Part model, mm, in its own coordinate system. Face numbers are marked on the shaded views. A direction names the side the tool comes from. Give positions to 0.01 mm unless a question says otherwise; leave off trailing zeros. Write each loop counter-clockwise with the first axis right and the second up, starting at its lowest first coordinate (ties: lowest second). Pieces come first, ordered by that corner, then holes. Notation, with made-up numbers: M -34.75,-35.75 L -12.75,-35.75 A8 cw -12.75,-29.75 Z; hole C -22,41.25 d10. An arc over 180 degrees is marked long. Use CSV: the item, a comma, the result in double quotes. Start each with the question number.
Item 1: Mould opens along Y. For the marked faces 5, 6 and 7 say: released by +Y, released by -Y, zero draft, split by the parting line, or undercut.
Item 2: Drill centre lines: line 1 (Y direction, x = 21, z = -1.5); line 2 (Y direction, x = 14, z = -4.5); line 3 (Z direction, x = -1, y = 18.25). Where is each one in solid material? Low to high. Write a range as [from, to].
Item 3: Cut at C-C (y = 2.75). List the corners of the cut face in (x, z).
Item 4: Which spindle directions (+Z, -Z, +X, -X, +Y, -Y) get a long thin tool onto all of the face, cutting with end or side? Do the marked faces 1, 2, 3 and 4. Say none if no direction does.
Item 5: Cut at D-D (x = -7.5). List the corners of the cut face in (y, z).
Item 6: Cut at A-A (x = 21.5). List the corners of the cut face in (y, z).
Item 7: Pin check, flat tips, straight feed: pin 1 (0.5 mm diameter, centred on x = 36.5, z = -1.5, fed in from -Y); pin 2 (3 mm diameter, centred on x = 16, z = -7, fed in from -Y); pin 3 (4 mm diameter, centred on x = 3, y = 21.5, fed in from -Z). Stop position of each tip, or through.
Item 8: Cut at B-B (y = 18.25). List the corners of the cut face in (x, z), then the cut area to 3 significant figures.
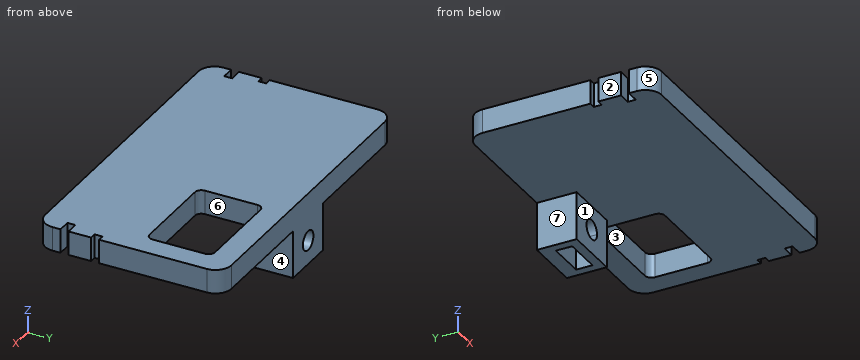
from build123d import *

# Parameters (mm, degrees)
BOSS_EXTRUDE1_DEPTH = 3.81
SKETCH2_W           = 8.89
SKETCH2_H           = 6.35
BOSS_EXTRUDE2_DEPTH = 7.62
CUT_EXTRUDE1_DEPTH  = 7.62
SKETCH4_W           = 6
SKETCH4_H           = 1.674510172
SKETCH4_H_2         = 0.925489708
CUT_EXTRUDE2_DEPTH  = 7.62


with BuildPart() as part:
    # Sketch1 → Boss-Extrude1 (new body)
    with BuildSketch(Plane.XY):
        with BuildLine():
            Line((37.128754647, 0.913367565), (37.128754647, 2.183367565))
            Line((37.128754647, 2.183367565), (35.096754647, 2.183367565))
            Line((35.096754647, 2.183367565), (35.096754647, 3.453367565))
            Line((35.096754647, 3.453367565), (37.128754647, 3.453367565))
            Line((37.128754647, 3.453367565), (37.128754647, 7.053367565))
            Line((37.128754647, 7.053367565), (36.112754647, 7.053367565))
            Line((36.112754647, 7.053367565), (36.112754647, 8.323367565))
            Line((36.112754647, 8.323367565), (37.128754647, 8.323367565))
            Line((37.128754647, 8.323367565), (37.128754647, 25.468367565))
            ThreePointArc((37.128754647, 25.468367565), (36.384805872, 27.264418789), (34.588754647, 28.008367565))
            Line((34.588754647, 28.008367565), (-10.750245353, 28.008367565))
            ThreePointArc((-10.750245353, 28.008367565), (-12.546296577, 27.264418789), (-13.290245353, 25.468367565))
            Line((-13.290245353, 25.468367565), (-13.290245353, 8.323367565))
            Line((-13.290245353, 8.323367565), (-12.274245353, 8.323367565))
            Line((-12.274245353, 8.323367565), (-12.274245353, 7.053367565))
            Line((-12.274245353, 7.053367565), (-13.290245353, 7.053367565))
            Line((-13.290245353, 7.053367565), (-13.290245353, 3.453367565))
            Line((-13.290245353, 3.453367565), (-11.258245353, 3.453367565))
            Line((-11.258245353, 3.453367565), (-11.258245353, 2.183367565))
            Line((-11.258245353, 2.183367565), (-13.290245353, 2.183367565))
            Line((-13.290245353, 2.183367565), (-13.290245353, 0.913367565))
            ThreePointArc((-13.290245353, 0.913367565), (-12.546296577, -0.882683659), (-10.750245353, -1.626632435))
            Line((-10.750245353, -1.626632435), (34.588754647, -1.626632435))
            ThreePointArc((34.588754647, -1.626632435), (36.384805872, -0.882683659), (37.128754647, 0.913367565))
        make_face()
        with BuildLine():
            Line((32.505954647, 24.279567565), (19.094754647, 24.279567565))
            ThreePointArc((19.094754647, 24.279567565), (18.376334158, 23.981988055), (18.078754647, 23.263567565))
            Line((18.078754647, 23.263567565), (18.078754647, 14.881567565))
            ThreePointArc((18.078754647, 14.881567565), (18.376334158, 14.163147076), (19.094754647, 13.865567565))
            Line((19.094754647, 13.865567565), (32.505954647, 13.865567565))
            ThreePointArc((32.505954647, 13.865567565), (33.224375137, 14.163147076), (33.521954647, 14.881567565))
            Line((33.521954647, 14.881567565), (33.521954647, 23.263567565))
            ThreePointArc((33.521954647, 23.263567565), (33.224375137, 23.981988055), (32.505954647, 24.279567565))
        make_face(mode=Mode.SUBTRACT)
    extrude(amount=-BOSS_EXTRUDE1_DEPTH)

    # Sketch2 → Boss-Extrude2 (add)
    with BuildSketch(Plane(origin=(0, 0, -3.81), x_dir=(-1, 0, 0), z_dir=(0, 0, -1))):
        with Locations((-11.919254647, 24.833367565)):
            Rectangle(SKETCH2_W, SKETCH2_H)
    extrude(amount=BOSS_EXTRUDE2_DEPTH)

    # Sketch3 → Cut-Extrude1 (cut)
    with BuildSketch(Plane(origin=(0, 28.008367565, 0), x_dir=(1, 0, 0), z_dir=(0, 1, 0))):
        with BuildLine():
            ThreePointArc((13.096102381, 8.628726629), (10.910528019, 8.796847734), (10.742406914, 6.611273371))
            Line((10.742406914, 6.611273371), (13.096102381, 8.628726629))
        make_face()
        with BuildLine():
            Line((13.096102381, 8.628726629), (10.742406914, 6.611273371))
            ThreePointArc((10.742406914, 6.611273371), (12.457021331, 6.166278227), (13.469254647, 7.62))
            ThreePointArc((13.469254647, 7.62), (13.372976421, 8.157766684), (13.096102381, 8.628726629))
        make_face()
    extrude(amount=-CUT_EXTRUDE1_DEPTH, mode=Mode.SUBTRACT)

    # Sketch4 → Cut-Extrude2 (cut)
    with BuildSketch(Plane(origin=(0, 0, -11.43), x_dir=(-1, 0, 0), z_dir=(0, 0, -1))):
        with Locations((-11.919254647, 23.996112479)):
            Rectangle(SKETCH4_W, SKETCH4_H)
        with Locations((-11.919254647, 25.296112419)):
            Rectangle(SKETCH4_W, SKETCH4_H_2)
    extrude(amount=-CUT_EXTRUDE2_DEPTH, mode=Mode.SUBTRACT)


solid = part.part
Worked answers:
1,face 5,"released by -Y"
1,face 6,"undercut"
1,face 7,"zero draft"
2,line 1,"y = [-1.63, 13.87], [24.28, 28.01]"
2,line 2,"y = [21.66, 23.16], [25.76, 28.01]"
2,line 3,"z = [-3.81, 0]"
3,outline,"M -11.26,-3.81 L 35.1,-3.81 L 35.1,0 L -11.26,0 Z"
4,face 1,"-Z, +X, -X, -Y"
4,face 2,"+Z, -Z, -X, +Y, -Y"
4,face 3,"+Z, -Z"
4,face 4,"-Z, +X, +Y, -Y"
5,outline,"M -1.63,-3.81 L 28.01,-3.81 L 28.01,0 L -1.63,0 Z"
6,outline,"M -1.63,-3.81 L 13.87,-3.81 L 13.87,0 L -1.63,0 Z; M 24.28,-3.81 L 28.01,-3.81 L 28.01,0 L 24.28,0 Z"
7,pin 1,"stops at y = -1.01"
7,pin 2,"stops at y = 21.66"
7,pin 3,"stops at z = -3.81"
8,outline,"M -13.29,-3.81 L 18.08,-3.81 L 18.08,0 L -13.29,0 Z; M 33.52,-3.81 L 37.13,-3.81 L 37.13,0 L 33.52,0 Z"
8,area,"133 mm^2"
